Job drawing, mm, ordinate dimensions from the low corner. One solid piece. A direction names the side the tool comes from. Coordinates: 2 decimals unless noted, no trailing zeros. Write each loop counter-clockwise with the first axis right and the second up, starting at its lowest first coordinate (ties: lowest second). Pieces come first, ordered by that corner, then holes.
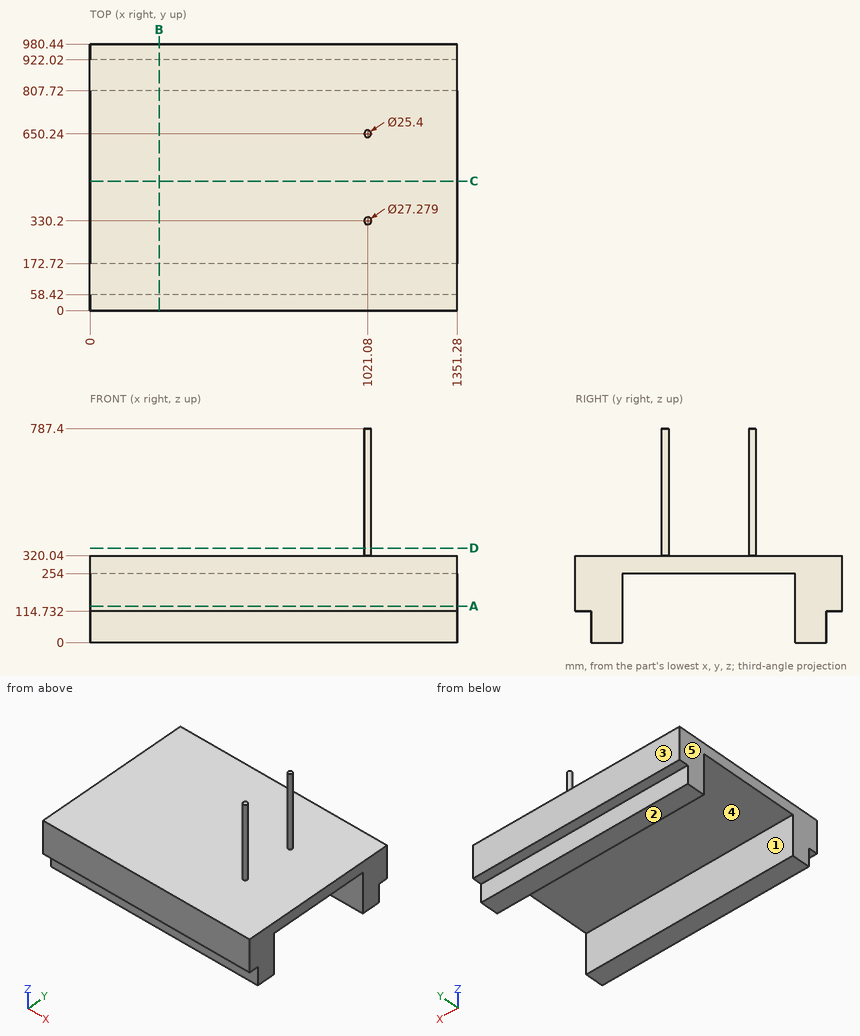
1. Saw through at D-D on z = 347.5. List the corners of the cut face in (x, y).
Computed values:
outline: circle Ø27.28 at (1021.08, 330.2); circle Ø25.4 at (1021.08, 650.24)
2. Flat gauge pins, fed straight in: pin 1 (3 mm diameter, centred on x = 394, y = 755.5, fed in from +Z); pin 2 (1.5 mm diameter, centred on x = 750, y = 566, fed in from -Z). Where does each tip first touch, or does it go through?
Computed values:
pin 1: stops at z = 320.04
pin 2: stops at z = 254
3. Saw through at B-B on x = 254. List the corners of the cut face in (y, z).
Computed values:
outline: (0, 114.73) - (58.42, 114.73) - (58.42, 0) - (172.72, 0) - (172.72, 254) - (807.72, 254) - (807.72, 0) - (922.02, 0) - (922.02, 114.73) - (980.44, 114.73) - (980.44, 320.04) - (0, 320.04) - close
4. Saw through at C-C on y = 476. List the corners of the cut face in (x, z).
Computed values:
outline: (0, 254) - (1351.28, 254) - (1351.28, 320.04) - (0, 320.04) - close
5. Mould opens along Y. For the marked faces 3, 4 and 5 say: +Y half, -Y half, draft (parallel to the pull), parting line (faces both ways), or undercut.
Computed values:
face 3: +Y half
face 4: undercut
face 5: draft
6. Saw through at A-A on z = 134. List the corners of the cut face in (x, y), plus the area to 3 significant figures.
Computed values:
outline: (0, 0) - (1351.28, 0) - (1351.28, 172.72) - (0, 172.72) - close; (0, 807.72) - (1351.28, 807.72) - (1351.28, 980.44) - (0, 980.44) - close
area: 467,000 mm2
7. Probe line 1 along Y through (x, z) = (76.5, 239); line 2 along Y through (x, z) = (1137.5, 38); line 3 along Z through (x, y) = (1047, 925). List the from-to ranges inside material, lowest first.
Computed values:
line 1: y = 0 to 172.72, 807.72 to 980.44
line 2: y = 58.42 to 172.72, 807.72 to 922.02
line 3: z = 114.73 to 320.04
8. 3-axis set-ups, long thin cutter, end or side, ignore diameter. For the marked faces 1 and 2: which of +Z, -Z, +X, -X, +Y, -Y reach the whole face in a straight line?
Computed values:
face 1: -Z, +X, -X
face 2: -Z, +X, -X, +Y, -Y
